from build123d import *

# Parameters (mm, degrees)
ESQUISSE1_W        = 95.5
ESQUISSE1_H        = 61
BOSS_EXTRU_1_DEPTH = 4
ESQUISSE2_W        = 108.5
ESQUISSE2_H        = 62
BOSS_EXTRU_2_DEPTH = 1.5
ESQUISSE3_W        = 2.5
ESQUISSE3_H        = 35.5
BOSS_EXTRU_3_DEPTH = 3
ESQUISSE4_W        = 0.65
ESQUISSE4_H        = 0.65
BOSS_EXTRU_4_DEPTH = 5.5


with BuildPart() as part:
    # Esquisse1 → Boss.-Extru.1 (new body)
    with BuildSketch(Plane.XY):
        Rectangle(ESQUISSE1_W, ESQUISSE1_H)
    extrude(amount=BOSS_EXTRU_1_DEPTH)

    # Esquisse2 → Boss.-Extru.2 (add)
    with BuildSketch(Plane(origin=(0, 0, 0), x_dir=(-1, 0, 0), z_dir=(0, 0, -1))):
        Rectangle(ESQUISSE2_W, ESQUISSE2_H)
    extrude(amount=BOSS_EXTRU_2_DEPTH)

    # Esquisse3 → Boss.-Extru.3 (add)
    with BuildSketch(Plane(origin=(0, 0, -1.5), x_dir=(-1, 0, 0), z_dir=(0, 0, -1))):
        with Locations((52.5, 0)):
            Rectangle(ESQUISSE3_W, ESQUISSE3_H)
    extrude(amount=BOSS_EXTRU_3_DEPTH)

    # Esquisse4 → Boss.-Extru.4 (add)
    with BuildSketch(Plane(origin=(0, 0, -4.5), x_dir=(-1, 0, 0), z_dir=(0, 0, -1))):
        with Locations((52.5, 16.775)):
            Rectangle(ESQUISSE4_W, ESQUISSE4_H)
        with Locations((52.5, 14.275)):
            Rectangle(ESQUISSE4_W, ESQUISSE4_H)
        with Locations((52.5, 11.775)):
            Rectangle(ESQUISSE4_W, ESQUISSE4_H)
        with Locations((52.5, 9.275)):
            Rectangle(ESQUISSE4_W, ESQUISSE4_H)
        with Locations((52.5, 6.775)):
            Rectangle(ESQUISSE4_W, ESQUISSE4_H)
        with Locations((52.5, 4.275)):
            Rectangle(ESQUISSE4_W, ESQUISSE4_H)
        with Locations((52.5, 1.775)):
            Rectangle(ESQUISSE4_W, ESQUISSE4_H)
        with Locations((52.5, -0.725)):
            Rectangle(ESQUISSE4_W, ESQUISSE4_H)
        with Locations((52.5, -3.225)):
            Rectangle(ESQUISSE4_W, ESQUISSE4_H)
        with Locations((52.5, -5.725)):
            Rectangle(ESQUISSE4_W, ESQUISSE4_H)
        with Locations((52.5, -8.225)):
            Rectangle(ESQUISSE4_W, ESQUISSE4_H)
        with Locations((52.5, -10.725)):
            Rectangle(ESQUISSE4_W, ESQUISSE4_H)
        with Locations((52.5, -13.225)):
            Rectangle(ESQUISSE4_W, ESQUISSE4_H)
        with Locations((52.5, -15.725)):
            Rectangle(ESQUISSE4_W, ESQUISSE4_H)
    extrude(amount=BOSS_EXTRU_4_DEPTH)


solid = part.part
Work out the finished part from the listing and answer in its coordinate system (mm). A direction names the side the tool comes from. Give positions to 0.01 mm unless a question says otherwise; leave off trailing zeros. Loops run counter-clockwise (first coordinate to the right, second up) from the corner with the lowest first, then second, coordinate; pieces in that order, holes last. Notation, with made-up numbers: M 37.25,71.25 L 64.25,71.25 A24 ccw 64.25,82.25 Z; hole C 87.25,7 d10. An arc over 180 degrees is marked long. Use CSV: the item, a comma, the result in double quotes.
1) Given P1, Ø0.5, axis at y = 9, z = -7, coming from the +X side (3 decimals); P2, Ø0.7, axis at x = -52.5, z = -6, coming from the +Y side; P3, Ø2, axis at x = -53, z = -3.5, coming from the +Y side, each flat-ended and moving along its own axis, determine where each tip first touches the part or whether it passes through.
Answer:
P1,"x = -52.175"
P2,"y = 17.1"
P3,"y = 17.75"
2) Find section B-B on z = -2.75. Write down the section's boundary in (x, y).
Answer:
outline,"M -53.75,-17.75 L -51.25,-17.75 L -51.25,17.75 L -53.75,17.75 Z"
3) Which of the six approach directions +Z, -Z, +X, -X, +Y, -Y give full straight-line access (tool end or side, diameter ignored) to faces 1 (the flat face through (-52, -17.75, -3)), 2 (the flat face through (47.75, 0, 2)), 3 (the flat face through (-52, 17.75, -3))?
Answer:
face 1,"-Z, +X, -X, -Y"
face 2,"+Z, +X, +Y, -Y"
face 3,"-Z, +X, -X, +Y"
4) Find section C-C on z = 2. Write down the section's boundary in (x, y), plus the area to 3 significant figures.
Answer:
outline,"M -47.75,-30.5 L 47.75,-30.5 L 47.75,30.5 L -47.75,30.5 Z"
area,"5,830 mm^2"
5) Find section A-A on x = -20. Write down the section's boundary in (y, z).
Answer:
outline,"M -31,-1.5 L 31,-1.5 L 31,0 L 30.5,0 L 30.5,4 L -30.5,4 L -30.5,0 L -31,0 Z"
6) Consider L1, parallel to Y at x = -2.5, z = 1; L2, parallel to X at y = -21, z = 3.5; L3, parallel to Z at x = -45.5, y = 16. Determine where each line is inside the solid, lowest interval first.
Answer:
L1,"-30.5 to 30.5"
L2,"-47.75 to 47.75"
L3,"-1.5 to 4"
